Geometry check sheet. Reference: drawing and pictorial views, mm from the part's lowest x, y, z. A direction names the side the tool comes from. Give positions to 0.01 mm unless a question says otherwise; leave off trailing zeros. Order: outer loops, then holes, each group sorted by start corner. A loop starts at its lowest first (then second) coordinate and runs counter-clockwise, first axis right, second up. Notation, with made-up numbers: (55.25, 72.25) -> (102.25, 72.25) arc R10 cw to (102.25, 85.25) -> close; hole circle Ø11 at (6.25, 17). An arc over 180 degrees is marked (long way). Write each question's results on one line, items separated by ' | '. Start each with the question number.
1. Mould release check, pull along X, two halves, no side actions. Record for the marked faces 5, 6 and 7: +X half, -X half, draft (parallel to the pull), parting line (faces both ways), or undercut.
2. Cross-section at B-B, the plane x = 830. Enter the section's corners in (y, z), then the cut area to 3 significant figures.
3. Set-up check for the marked faces 1, 2, 3 and 4: record each of +Z, -Z, +X, -X, +Y, -Y from which the full face is reachable in a straight line by a thin tool's end or side.
4. Depth check by flat-ended pin: pin 1 Ø5 at (x, z) = (95.5, 195) entering from -Y; pin 2 Ø3 at (y, z) = (26, 177) entering from +X; pin 3 Ø2 at (y, z) = (50, 135) entering from +X. Enter the tip coordinate at first touch or a pass-through.
5. Material ranges on L1, parallel to X at y = 70, z = 150; L2, parallel to X at y = 130.5, z = 153.5; L3, parallel to Z at x = 830, y = 215, recorded low to high. Write a range as from..to.
6. Cross-section at C-C, the plane x = 475. Enter the section's corners in (y, z).
7. Cross-section at D-D, the plane z = 150. State how many separate pieces and enclosed holes the cut face has, then the cut area to 3 significant figures.
8. Cross-section at A-A, the plane y = 121.5. Enter the section's corners in (x, z).
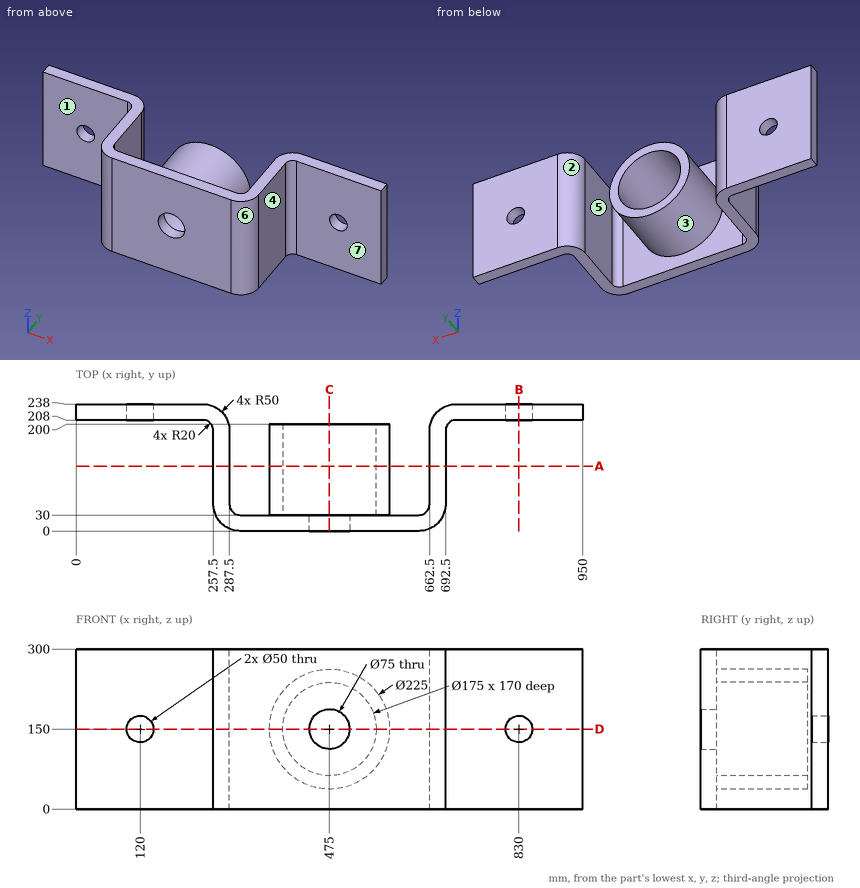
Results below:
1) face 5: undercut | face 6: +X half | face 7: draft
2) outline: (208, 0) -> (238, 0) -> (238, 125) -> (208, 125) -> close; (208, 175) -> (238, 175) -> (238, 300) -> (208, 300) -> close | area: 7,500 mm²
3) face 1: +Z, -Z, -X, -Y | face 2: +Z, -Z, +Y | face 3: +Y | face 4: +Z, -Z, +X, -Y
4) pin 1: stops at y = 208 | pin 2: stops at x = 687.15 | pin 3: stops at x = 692.5
5) L1: x = 257.5..287.5, 362.5..387.5, 562.5..587.5, 662.5..692.5 | L2: x = 257.5..287.5, 362.55..387.57, 562.43..587.45, 662.5..692.5 | L3: z = 0..125, 175..300
6) outline: (0, 0) -> (30, 0) -> (30, 37.5) -> (200, 37.5) -> (200, 62.5) -> (30, 62.5) -> (30, 112.5) -> (0, 112.5) -> close; (0, 187.5) -> (30, 187.5) -> (30, 237.5) -> (200, 237.5) -> (200, 262.5) -> (30, 262.5) -> (30, 300) -> (0, 300) -> close
7) separate pieces: 4 | enclosed holes: 0 | area: 42,400 mm²
8) outline: (257.5, 0) -> (287.5, 0) -> (287.5, 300) -> (257.5, 300) -> close; circle Ø225 at (475, 150); (662.5, 0) -> (692.5, 0) -> (692.5, 300) -> (662.5, 300) -> close; hole circle Ø175 at (475, 150)
